Here's how the part is built. I have some questions about the finished solid (model axes, mm). Face numbers are marked on the shaded views. A direction names the side the tool comes from. Give positions to 0.01 mm unless a question says otherwise; leave off trailing zeros. Write each loop counter-clockwise with the first axis right and the second up, starting at its lowest first coordinate (ties: lowest second). Pieces come first, ordered by that corner, then holes. Notation, with made-up numbers: M 88.25,13 L 97.25,13 A11 ccw 97.25,31 Z; hole C -24,-18.5 d6. An arc over 180 degrees is marked long. Answer as CSV lines item,"result". Start each with the question number.
Q1. Suppose I cut it at C-C (y = 0). Write out the boundary of the cut face in (x, z).
Q2. Suppose I cut it at A-A (z = -306). Write out the boundary of the cut face in (x, y).
Q3. For pin 1 (3 mm diameter, centred on y = -84.5, z = -62, fed in from +X); pin 2 (1.5 mm diameter, centred on y = -28.5, z = -300.5, fed in from -X); pin 3 (4 mm diameter, centred on x = -56.5, z = -224, fed in from -Y), each with a flat end and sliding along its axis, tell me the tip position at first contact or that it passes through.
Q4. If I drill on line 1 along Z through (x, y) = (-99, 8); line 2 along Z through (x, y) = (-9.5, 18); line 3 along Y through (x, z) = (-96, -344), over which ranges is the centre line in solid material (lowest first)?
Q5. On a 3-axis mill with a long thin cutter (end or side, diameter ignored), from which of +Z, -Z, +X, -X, +Y, -Y can I reach the whole of each face in a straight line? I mean the marked faces 4 and 5. Say none if no direction works.
Q6. Thinking about a two-plate mould opening in Y: for the marked faces 1, 2 and 3, which applies, +Y half, -Y half, draft (parallel to the pull), parting line (faces both ways), or undercut?
Q7. Suppose I cut it at B-B (x = -77). Write out the boundary of the cut face in (y, z).
Q8. Suppose I cut it at D-D (x = -50). Write out the boundary of the cut face in (y, z), then the cut area to 3 significant figures.
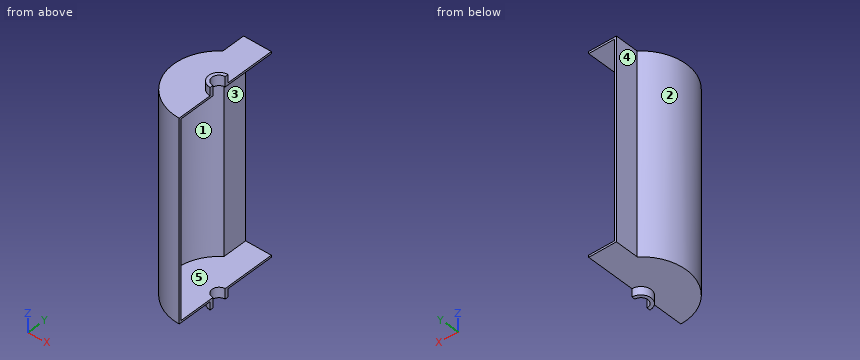
```python
from build123d import *

# Parameters (mm, degrees)
BOSS_EXTRUDE1_DEPTH      = 20
BOSS_EXTRUDE1_DEPTH_BACK = 5
BOSS_EXTRUDE2_START      = -5
BOSS_EXTRUDE2_DEPTH      = 5
BOSS_EXTRUDE3_REACH      = 541.227


with BuildPart() as part:
    # Sketch1 → Boss-Extrude1 (new, two sides: drawn at the far end of the back side and taken through both)
    with BuildSketch(Plane.XY.offset(-BOSS_EXTRUDE1_DEPTH_BACK)):
        with BuildLine():
            Line((0, 25), (0, 17))
            ThreePointArc((0, 17), (-17, 0), (0, -17))
            Line((0, -17), (0, -25))
            ThreePointArc((0, -25), (-25, 0), (0, 25))
        make_face()
    extrude(amount=BOSS_EXTRUDE1_DEPTH + BOSS_EXTRUDE1_DEPTH_BACK)

    # Sketch2 → Boss-Extrude2 (add)
    with BuildSketch(Plane.XY.offset(BOSS_EXTRUDE2_START)):
        with BuildLine():
            Line((0, 25), (0, 146.014758251))
            Line((0, 146.014758251), (-68.093579632, 146.014758251))
            Line((-68.093579632, 146.014758251), (-68.093579632, 88.087940795))
            ThreePointArc((-68.093579632, 88.087940795), (-105.365516189, -35.976782774), (0, -111.338317306))
            Line((0, -111.338317306), (0, -25))
            ThreePointArc((0, -25), (-25, 0), (0, 25))
        make_face()
    extrude(amount=BOSS_EXTRUDE2_DEPTH)


with BuildPart() as body_2:
    # Mirror2: mirrored copy
    add(part.part.mirror(Plane.XY.offset(-246)))

    # Sketch3 → Boss-Extrude3 (add, up to next)
    with BuildSketch(Plane(origin=(0, 0, -5), x_dir=(-1, 0, 0), z_dir=(0, 0, -1)), mode=Mode.PRIVATE) as boss_extrude3_sk1:
        with BuildLine():
            Line((68.093579632, 146.014758251), (68.093579632, 88.087940795))
            ThreePointArc((68.093579632, 88.087940795), (105.365516189, -35.976782774), (0, -111.338317306))
            Line((0, -111.338317306), (0, -106.338317306))
            ThreePointArc((0, -106.338317306), (101.020289155, -33.207512802), (63.093579632, 85.598118769))
            Line((63.093579632, 85.598118769), (63.093579632, 146.014758251))
            Line((63.093579632, 146.014758251), (68.093579632, 146.014758251))
        make_face()
    boss_extrude3_tool1 = extrude(boss_extrude3_sk1.sketch, amount=BOSS_EXTRUDE3_REACH, mode=Mode.PRIVATE) - body_2.part

    add(part.part)  # Boss-Extrude3 merges part
    add(boss_extrude3_tool1.solids().sort_by_distance((-65.897627, 115.806439, -5))[0])


solid = body_2.part
```
Resolved:
1,outline,"M -111.34,-492 L -25,-492 L -25,-512 L -17,-512 L -17,-487 L -106.34,-487 L -106.34,-5 L -17,-5 L -17,20 L -25,20 L -25,0 L -111.34,0 Z"
2,outline,"M -68.09,88.09 A111.34 ccw 0,-111.34 L 0,-106.34 A106.34 cw -63.09,85.6 L -63.09,146.01 L -68.09,146.01 Z"
3,pin 1,"x = -62.54"
3,pin 2,"x = -107.82"
3,pin 3,"y = -97.09"
4,line 1,"-492 to -487, -5 to 0"
4,line 2,"-512 to -487, -5 to 20"
4,line 3,"-56.39 to -45.74, 45.74 to 56.39"
5,face 4,"+Z, -Z, -X, +Y"
5,face 5,"+X"
6,face 1,"undercut"
6,face 2,"parting line"
6,face 3,"draft"
7,outline,"M -80.42,-492 L 80.42,-492 L 80.42,0 L -80.42,0 Z; hole M -73.34,-487 L 73.34,-487 L 73.34,-5 L -73.34,-5 Z"
8,outline,"M -99.48,-492 L 146.01,-492 L 146.01,-487 L -93.85,-487 L -93.85,-5 L 146.01,-5 L 146.01,0 L -99.48,0 Z"
8,area,"5,170 mm^2"
